Job drawing, mm, ordinate dimensions from the low corner. One solid piece. A direction names the side the tool comes from. Round coordinates to 2 decimals unless told otherwise and drop trailing zeros. Loops run counter-clockwise (first coordinate to the right, second up) from the corner with the lowest first, then second, coordinate; pieces in that order, holes last. Notation, with made-up numbers: (-4.5, 57.5) - (2.5, 57.5) arc R29 cw to (2.5, 86.5) - close; hole circle Ø9 at (45.25, -7). An arc over 180 degrees is marked (long way). One line per question, with ' | ' between items. Start each with the question number.
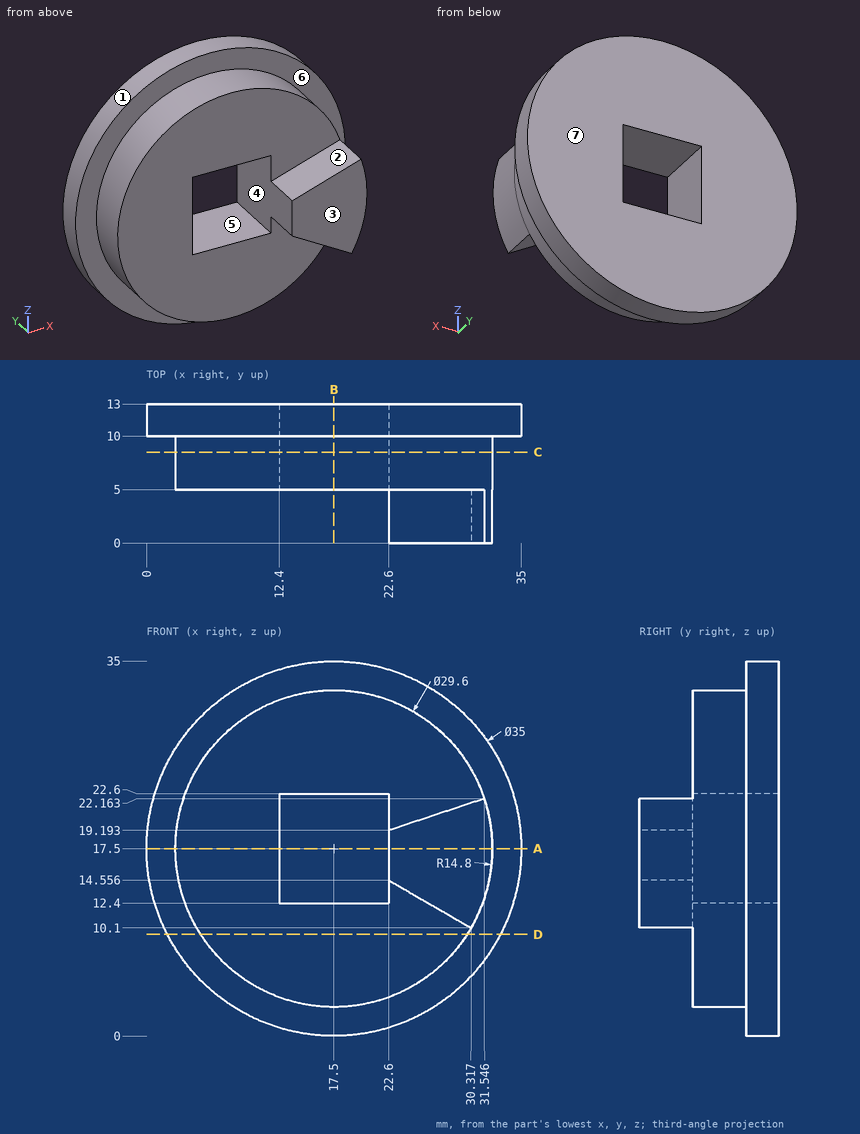
1) Saw through at C-C on y = 8.5. Write the cut outline in (x, z), and give its area (3 significant figures).
2) Saw through at A-A on z = 17.5. Write the cut outline in (x, y).
3) Saw through at D-D on z = 9.5. Write the cut outline in (x, y) (1 decimal), and give its area (3 significant figures).
4) Wall check: line 1 (Y direction, x = 20, z = 7.5); line 2 (Y direction, x = 6, z = 8); line 3 (X direction, y = 10.25, z = 16.5). Give the ranges that are in metal, low to high. Write a range as [from, to].
5) Two-plate mould, pull along X, no slides. Class the marked faces 1, 2, 3 and 4: +X half, -X half, draft (parallel to the pull), parting line (faces both ways), or undercut.
6) Drop flat-ended pins along their axis: pin 1 (5 mm diameter, centred on x = 31.5, y = 9.5, fed in from +Z) (1 decimal); pin 2 (5 mm diameter, centred on x = 19, z = 3.5, fed in from -Y); pin 3 (1.5 mm diameter, centred on x = 26, y = 7.5, fed in from -Z). Give the stop position or say it passes through.
7) Saw through at B-B on x = 17.5. Write the cut outline in (y, z).
8) Tool access for the marked faces 5, 6 and 7: list every direction of +Z, -Z, +X, -X, +Y, -Y with a clear straight run to the whole face (end or side of a thin tool).
Answer key:
1) outline: circle Ø29.6 at (17.5, 17.5); hole (12.4, 12.4) - (22.6, 12.4) - (22.6, 22.6) - (12.4, 22.6) - close | area: 584 mm²
2) outline: (0, 10) - (2.7, 10) - (2.7, 5) - (12.4, 5) - (12.4, 13) - (0, 13) - close; (22.6, 0) - (32.3, 0) - (32.3, 10) - (35, 10) - (35, 13) - (22.6, 13) - close
3) outline: (1.9, 10) - (5, 10) - (5, 5) - (30, 5) - (30, 10) - (33.1, 10) - (33.1, 13) - (1.9, 13) - close | area: 218 mm²
4) line 1: [5, 13] | line 2: [10, 13] | line 3: [0.03, 12.4], [22.6, 34.97]
5) face 1: parting line | face 2: -X half | face 3: draft | face 4: undercut
6) pin 1: z = 30.6 | pin 2: y = 5 | pin 3: z = 4.89
7) outline: (5, 2.7) - (10, 2.7) - (10, 0) - (13, 0) - (13, 12.4) - (5, 12.4) - close; (5, 22.6) - (13, 22.6) - (13, 35) - (10, 35) - (10, 32.3) - (5, 32.3) - close
8) face 5: +Y, -Y | face 6: -Y | face 7: +Z, -Z, +X, -X, +Y
